Here's how the part is built. I have some questions about the finished solid (model axes, mm). Face numbers are marked on the shaded views. A direction names the side the tool comes from. Round coordinates to 2 decimals unless told otherwise and drop trailing zeros. Write each loop counter-clockwise with the first axis right and the second up, starting at its lowest first coordinate (ties: lowest second). Pieces come first, ordered by that corner, then holes. Notation, with made-up numbers: M -35,0 L 0,0 A18 ccw 0,26 Z; hole C 39,46.25 d11. An arc over 180 degrees is marked long. Use a Markdown table: item, result. Add a question column.
```python
from build123d import *

# Parameters (mm, degrees)
BOSS_EXTRUDE1_DEPTH = 80
SHELL1_T            = -3
SKETCH3_W           = 46
SKETCH3_H           = 47
BOSS_EXTRUDE2_DEPTH = 17
SKETCH4_W           = 10.2
SKETCH4_H           = 10.2
CUT_EXTRUDE1_DEPTH  = 20
SKETCH6_W           = 15
SKETCH6_H           = 12.8
CUT_EXTRUDE2_DEPTH  = 3
SKETCH7_W           = 40.4
SKETCH7_H           = 50
CUT_EXTRUDE3_DEPTH  = 5
FILLET1_R           = 4
CUT_EXTRUDE7_DEPTH  = 47
SKETCH13_R          = 1.5
CUT_EXTRUDE8_DEPTH  = 25
SKETCH14_R          = 3.1
CUT_EXTRUDE9_DEPTH  = 2
SKETCH17_W          = 45
SKETCH17_H          = 5
BOSS_EXTRUDE5_DEPTH = 74
CUT_EXTRUDE10_REACH = 126.093
SKETCH18_W          = 54
SKETCH18_H          = 45
CUT_EXTRUDE11_REACH = 126.093
SKETCH19_R          = 1.45
BOSS_EXTRUDE6_DEPTH = 47
SKETCH22_R          = 1.45
CUT_EXTRUDE12_DEPTH = 135.415364765
CUT_EXTRUDE13_REACH = 126.857
SKETCH24_R          = 3.7
SKETCH24_W          = 2
SKETCH24_H          = 3
BOSS_EXTRUDE7_DEPTH = 74
SKETCH27_R          = 1.65
CUT_EXTRUDE14_DEPTH = 10
CUT_EXTRUDE15_START = -3
CUT_EXTRUDE15_DEPTH = 32
CUT_EXTRUDE16_DEPTH = 30
BOSS_EXTRUDE8_DEPTH = 20
SKETCH31_R          = 1.5
CUT_EXTRUDE17_DEPTH = 123.649786567
CUT_EXTRUDE18_DEPTH = 15
CUT_EXTRUDE19_REACH = 126.093
SKETCH33_W          = 10
SKETCH33_H          = 5
SKETCH34_R          = 1.6
CUT_EXTRUDE20_DEPTH = 135.415364765
CUT_EXTRUDE22_DEPTH = 14
CUT_EXTRUDE23_REACH = 126.857
SKETCH37_R          = 3.2
SKETCH38_W          = 10
SKETCH38_H          = 18.980735551
SKETCH38_R          = 3.2
BOSS_EXTRUDE9_DEPTH = 3


with BuildPart() as part:
    # Sketch2 → Boss-Extrude1 (new body)
    with BuildSketch(Plane(origin=(0, 0, 0), x_dir=(0, 0, -1), z_dir=(1, 0, 0))):
        Polygon((-27.320490368, 20.998248687), (-27.320490368, -29.001751313), (12.679509632, -29.001751313), (12.679509632, -48.511383538), (27.679509632, -48.511383538), (82.679509632, 0.998248687), (82.679509632, 20.998248687), align=None)
    extrude(amount=BOSS_EXTRUDE1_DEPTH)

    # Shell1
    shell1_openings = [part.faces().sort_by_distance(p)[0] for p in [
        (40, 20.998248687, -27.679509632),
    ]]
    offset(amount=SHELL1_T, openings=shell1_openings, kind=Kind.INTERSECTION)

    # Sketch3 → Boss-Extrude2 (add)
    with BuildSketch(Plane(origin=(0, 0, 24.320490368), x_dir=(-1, 0, 0), z_dir=(0, 0, -1))):
        with Locations((-40, -2.501751313)):
            Rectangle(SKETCH3_W, SKETCH3_H)
    extrude(amount=BOSS_EXTRUDE2_DEPTH)

    # Sketch4 → Cut-Extrude1 (cut)
    with BuildSketch(Plane.XY.offset(27.320490368)):
        with Locations((40, -4.001751313)):
            Rectangle(SKETCH4_W, SKETCH4_H)
    extrude(amount=-CUT_EXTRUDE1_DEPTH, mode=Mode.SUBTRACT)

    # Sketch6 → Cut-Extrude2 (cut)
    with BuildSketch(Plane.XZ.offset(29.001751313)):
        with Locations((51.5, 0.920490368)):
            Rectangle(SKETCH6_W, SKETCH6_H)
        with Locations((28.5, 0.920490368)):
            Rectangle(SKETCH6_W, SKETCH6_H)
    extrude(amount=-CUT_EXTRUDE2_DEPTH, mode=Mode.SUBTRACT)

    # Sketch7 → Cut-Extrude3 (cut)
    with BuildSketch(Plane.XY.offset(27.320490368)):
        with Locations((40, -4.001751313)):
            Rectangle(SKETCH7_W, SKETCH7_H)
    extrude(amount=-CUT_EXTRUDE3_DEPTH, mode=Mode.SUBTRACT)

    # Fillet1
    fillet1_edges = [part.edges().sort_by_distance(p)[0] for p in [
        (19.8, -4.001751313, 27.320490368),
        (60.2, -4.001751313, 27.320490368),
        (80, -4.001751313, 27.320490368),
        (0, -4.001751313, 27.320490368),
    ]]
    fillet(fillet1_edges, radius=FILLET1_R)

    # Sketch12 → Cut-Extrude7 (cut)
    with BuildSketch(Plane(origin=(0, 20.998248687, 0), x_dir=(1, 0, 0), z_dir=(0, 1, 0))):
        Polygon((33, -7.320490368), (19.8, -12.320490368), (17, -24.320490368), (17, -7.320490368), align=None)
        Polygon((47, -7.320490368), (63, -7.320490368), (63, -24.320490368), (60.2, -12.320490368), align=None)
    extrude(amount=-CUT_EXTRUDE7_DEPTH, mode=Mode.SUBTRACT)

    # Sketch13 → Cut-Extrude8 (cut)
    with BuildSketch(Plane(origin=(0, 20.998248687, 0), x_dir=(1, 0, 0), z_dir=(0, 1, 0))):
        with Locations(Location((26, -17.320490368, 0), (0, 0, 270))):
            Circle(SKETCH13_R)
        with Locations(Location((54, -17.320490368, 0), (0, 0, 270))):
            Circle(SKETCH13_R)
    extrude(amount=-CUT_EXTRUDE8_DEPTH, mode=Mode.SUBTRACT)

    # Sketch14 → Cut-Extrude9 (cut)
    with BuildSketch(Plane(origin=(0, 20.998248687, 0), x_dir=(1, 0, 0), z_dir=(0, 1, 0))):
        with Locations(Location((26, -17.320490368, 0), (0, 0, 270))):
            Circle(SKETCH14_R)
        with Locations(Location((54, -17.320490368, 0), (0, 0, 270))):
            Circle(SKETCH14_R)
    extrude(amount=-CUT_EXTRUDE9_DEPTH, mode=Mode.SUBTRACT)

    # Sketch17 → Boss-Extrude5 (add)
    with BuildSketch(Plane.ZY.offset(-77)):
        with Locations((-23.179509632, -4.501751313)):
            Rectangle(SKETCH17_W, SKETCH17_H)
    extrude(amount=BOSS_EXTRUDE5_DEPTH)

    # Sketch18 → Cut-Extrude10 (cut, up to next)
    with BuildSketch(Plane(origin=(0, -2.001751313, 0), x_dir=(1, 0, 0), z_dir=(0, 1, 0)), mode=Mode.PRIVATE) as cut_extrude10_sk1:
        with Locations((40, 23.179509632)):
            Rectangle(SKETCH18_W, SKETCH18_H)
    cut_extrude10_tool1 = extrude(cut_extrude10_sk1.sketch, amount=-CUT_EXTRUDE10_REACH, mode=Mode.PRIVATE) & part.part
    add(cut_extrude10_tool1.solids().sort_by_distance((40, -2.001751, -23.17951))[0], mode=Mode.SUBTRACT)

    # Sketch19 → Cut-Extrude11 (cut, up to next)
    with BuildSketch(Plane(origin=(0, -2.001751313, 0), x_dir=(1, 0, 0), z_dir=(0, 1, 0)), mode=Mode.PRIVATE) as cut_extrude11_sk1:
        with Locations(Location((72, 37.179509632, 0), (0, 0, 270))):
            Circle(SKETCH19_R)
    cut_extrude11_tool1 = extrude(cut_extrude11_sk1.sketch, amount=-CUT_EXTRUDE11_REACH, mode=Mode.PRIVATE) & part.part
    # Sketch19 → Cut-Extrude11 (cut, up to next)
    with BuildSketch(Plane(origin=(0, -2.001751313, 0), x_dir=(1, 0, 0), z_dir=(0, 1, 0)), mode=Mode.PRIVATE) as cut_extrude11_sk2:
        with Locations(Location((72, 6.179509632, 0), (0, 0, 270))):
            Circle(SKETCH19_R)
    cut_extrude11_tool2 = extrude(cut_extrude11_sk2.sketch, amount=-CUT_EXTRUDE11_REACH, mode=Mode.PRIVATE) & part.part
    # Sketch19 → Cut-Extrude11 (cut, up to next)
    with BuildSketch(Plane(origin=(0, -2.001751313, 0), x_dir=(1, 0, 0), z_dir=(0, 1, 0)), mode=Mode.PRIVATE) as cut_extrude11_sk3:
        with Locations(Location((8, 33.179509632, 0), (0, 0, 270))):
            Circle(SKETCH19_R)
    cut_extrude11_tool3 = extrude(cut_extrude11_sk3.sketch, amount=-CUT_EXTRUDE11_REACH, mode=Mode.PRIVATE) & part.part
    # Sketch19 → Cut-Extrude11 (cut, up to next)
    with BuildSketch(Plane(origin=(0, -2.001751313, 0), x_dir=(1, 0, 0), z_dir=(0, 1, 0)), mode=Mode.PRIVATE) as cut_extrude11_sk4:
        with Locations(Location((8, 6.179509632, 0), (0, 0, 270))):
            Circle(SKETCH19_R)
    cut_extrude11_tool4 = extrude(cut_extrude11_sk4.sketch, amount=-CUT_EXTRUDE11_REACH, mode=Mode.PRIVATE) & part.part
    add(cut_extrude11_tool1.solids().sort_by_distance((72, -2.001751, -37.17951))[0], mode=Mode.SUBTRACT)
    add(cut_extrude11_tool2.solids().sort_by_distance((72, -2.001751, -6.17951))[0], mode=Mode.SUBTRACT)
    add(cut_extrude11_tool3.solids().sort_by_distance((8, -2.001751, -33.17951))[0], mode=Mode.SUBTRACT)
    add(cut_extrude11_tool4.solids().sort_by_distance((8, -2.001751, -6.17951))[0], mode=Mode.SUBTRACT)

    # Sketch21 → Boss-Extrude6 (add)
    with BuildSketch(Plane(origin=(0, -26.001751313, 0), x_dir=(1, 0, 0), z_dir=(0, 1, 0))):
        Polygon((3, -24.320490368), (3, -14.320490368), (19.333333333, -14.320490368), (17, -24.320490368), align=None)
    extrude(amount=BOSS_EXTRUDE6_DEPTH)

    # Sketch22 → Cut-Extrude12 (cut, through all)
    with BuildSketch(Plane(origin=(0, 20.998248687, 0), x_dir=(1, 0, 0), z_dir=(0, 1, 0))):
        with Locations(Location((10, -19.320490368, 0), (0, 0, 270))):
            Circle(SKETCH22_R)
    extrude(amount=-CUT_EXTRUDE12_DEPTH, mode=Mode.SUBTRACT)

    # Sketch24 → Cut-Extrude13 (cut, up to next)
    with BuildSketch(Plane(origin=(80, 0, 0), x_dir=(0, 0, -1), z_dir=(1, 0, 0)), mode=Mode.PRIVATE) as cut_extrude13_sk1:
        with Locations((26.679509632, -30.511383538)):
            Circle(SKETCH24_R)
    cut_extrude13_tool1 = extrude(cut_extrude13_sk1.sketch, amount=-CUT_EXTRUDE13_REACH, mode=Mode.PRIVATE) & part.part
    # Sketch24 → Cut-Extrude13 (cut, up to next)
    with BuildSketch(Plane(origin=(80, 0, 0), x_dir=(0, 0, -1), z_dir=(1, 0, 0)), mode=Mode.PRIVATE) as cut_extrude13_sk2:
        with Locations((34.379509632, -30.511383538)):
            Rectangle(SKETCH24_W, SKETCH24_H)
    cut_extrude13_tool2 = extrude(cut_extrude13_sk2.sketch, amount=-CUT_EXTRUDE13_REACH, mode=Mode.PRIVATE) & part.part
    add(cut_extrude13_tool1.solids().sort_by_distance((80, -30.511384, -26.67951))[0], mode=Mode.SUBTRACT)
    add(cut_extrude13_tool2.solids().sort_by_distance((80, -30.511384, -34.37951))[0], mode=Mode.SUBTRACT)

    # Sketch26 → Boss-Extrude7 (add)
    with BuildSketch(Plane(origin=(3, 0, 0), x_dir=(0, 0, -1), z_dir=(1, 0, 0))):
        Polygon((79.679509632, 2.334161996), (63.679509632, 2.334161996), (63.679509632, -12.068640106), align=None)
    extrude(amount=BOSS_EXTRUDE7_DEPTH)

    # Sketch27 → Cut-Extrude14 (cut)
    with BuildSketch(Plane(origin=(0, 2.334161996, 0), x_dir=(1, 0, 0), z_dir=(0, 1, 0))):
        with Locations(Location((6, 76.679509632, 0), (0, 0, 270))):
            Circle(SKETCH27_R)
        with Locations(Location((74, 76.679509632, 0), (0, 0, 270))):
            Circle(SKETCH27_R)
    extrude(amount=-CUT_EXTRUDE14_DEPTH, mode=Mode.SUBTRACT)

    # Sketch28 → Cut-Extrude15 (cut)
    with BuildSketch(Plane(origin=(0, 2.334161996, 0), x_dir=(1, 0, 0), z_dir=(0, 1, 0)).offset(CUT_EXTRUDE15_START)):
        Polygon((74, 79.929509632), (71.185417438, 78.304509632), (71.185417438, 75.054509632), (74, 73.429509632), (76.814582562, 75.054509632), (76.814582562, 78.304509632), align=None)
        Polygon((6, 73.429509632), (8.814582562, 75.054509632), (8.814582562, 78.304509632), (6, 79.929509632), (3.185417438, 78.304509632), (3.185417438, 75.054509632), align=None)
    extrude(amount=-CUT_EXTRUDE15_DEPTH, mode=Mode.SUBTRACT)

    # Sketch29 → Cut-Extrude16 (cut)
    with BuildSketch(Plane.XZ.offset(29.001751313)):
        Polygon((7.185417438, 17.695490368), (10, 16.070490368), (12.814582562, 17.695490368), (12.814582562, 20.945490368), (10, 22.570490368), (7.185417438, 20.945490368), align=None)
    extrude(amount=-CUT_EXTRUDE16_DEPTH, mode=Mode.SUBTRACT)

    # Sketch30 → Boss-Extrude8 (add)
    with BuildSketch(Plane(origin=(0, -26.001751313, 0), x_dir=(1, 0, 0), z_dir=(0, 1, 0))):
        Polygon((77, -24.320490368), (63, -24.320490368), (60.2, -12.320490368), (77, -12.320490368), align=None)
    extrude(amount=BOSS_EXTRUDE8_DEPTH)

    # Sketch31 → Cut-Extrude17 (cut, through all)
    with BuildSketch(Plane(origin=(0, -6.001751313, 0), x_dir=(1, 0, 0), z_dir=(0, 1, 0))):
        with Locations(Location((72, -21.320490368, 0), (0, 0, 270))):
            Circle(SKETCH31_R)
    extrude(amount=-CUT_EXTRUDE17_DEPTH, mode=Mode.SUBTRACT)

    # Sketch32 → Cut-Extrude18 (cut)
    with BuildSketch(Plane.XZ.offset(29.001751313)):
        Polygon((72, 24.570490368), (69.185417438, 22.945490368), (69.185417438, 19.695490368), (72, 18.070490368), (74.814582562, 19.695490368), (74.814582562, 22.945490368), align=None)
    extrude(amount=-CUT_EXTRUDE18_DEPTH, mode=Mode.SUBTRACT)

    # Sketch33 → Cut-Extrude19 (cut, up to next)
    with BuildSketch(Plane(origin=(0, -2.001751313, 0), x_dir=(1, 0, 0), z_dir=(0, 1, 0)), mode=Mode.PRIVATE) as cut_extrude19_sk1:
        with Locations((72, 43.179509632)):
            Rectangle(SKETCH33_W, SKETCH33_H)
    cut_extrude19_tool1 = extrude(cut_extrude19_sk1.sketch, amount=-CUT_EXTRUDE19_REACH, mode=Mode.PRIVATE) & part.part
    add(cut_extrude19_tool1.solids().sort_by_distance((72, -2.001751, -43.17951))[0], mode=Mode.SUBTRACT)

    # Sketch34 → Cut-Extrude20 (cut, through all)
    with BuildSketch(Plane(origin=(0, 20.998248687, 0), x_dir=(1, 0, 0), z_dir=(0, 1, 0))):
        with Locations(Location((40, -17.320490368, 0), (0, 0, 270))):
            Circle(SKETCH34_R)
    extrude(amount=-CUT_EXTRUDE20_DEPTH, mode=Mode.SUBTRACT)

    # Sketch36 → Cut-Extrude22 (cut)
    with BuildSketch(Plane.XZ.offset(29.001751313)):
        Polygon((38.375, 20.13507293), (36.75, 17.320490368), (38.375, 14.505907805), (41.625, 14.505907805), (43.25, 17.320490368), (41.625, 20.13507293), align=None)
    extrude(amount=-CUT_EXTRUDE22_DEPTH, mode=Mode.SUBTRACT)

    # Sketch37 → Cut-Extrude23 (cut, up to next)
    with BuildSketch(Plane(origin=(80, 0, 0), x_dir=(0, 0, -1), z_dir=(1, 0, 0)), mode=Mode.PRIVATE) as cut_extrude23_sk1:
        with Locations((-3.320490368, -16.511383538)):
            Circle(SKETCH37_R)
    cut_extrude23_tool1 = extrude(cut_extrude23_sk1.sketch, amount=-CUT_EXTRUDE23_REACH, mode=Mode.PRIVATE) & part.part
    add(cut_extrude23_tool1.solids().sort_by_distance((80, -16.511384, 3.32049))[0], mode=Mode.SUBTRACT)

    # Sketch38 → Boss-Extrude9 (add)
    with BuildSketch(Plane.ZY.offset(-77)):
        with Locations((3.320490368, -16.511383538)):
            Rectangle(SKETCH38_W, SKETCH38_H)
        with Locations(Location((3.320490368, -16.511383538, 0), (0, 0, 180))):
            Circle(SKETCH38_R, mode=Mode.SUBTRACT)
    extrude(amount=BOSS_EXTRUDE9_DEPTH)


solid = part.part
```
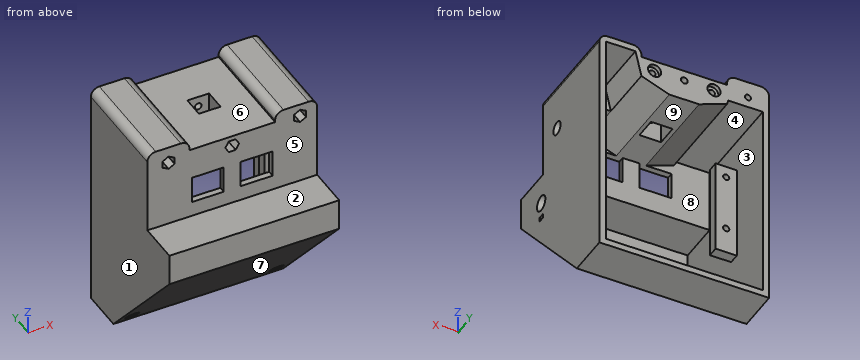
Item 1: Imagine slicing it at B-B on x = 26. List the corners of the cut face in (y, z) for me.
Item 2: Imagine slicing it at A-A on z = -3. List the corners of the cut face in (x, y) for me, plus the area to 3 significant figures.
Item 3: Imagine slicing it at C-C on y = 16. List the corners of the cut face in (x, z) for me.
Item 4: Imagine slicing it at D-D on x = 40. Count the separate pieces of the cut face and the enclosed holes in it, plus the area to 3 significant figures.
Item 5: For pin 1 Ø18.5 at (x, y) = (72.5, -12.5) entering from -Z; pin 2 Ø5 at (x, y) = (39.5, -27.5) entering from -Z; pin 3 Ø1.7 at (x, z) = (73.5, -75.5) entering from -Y; pin 4 Ø3 at (y, z) = (-29, -54.5) entering from +X, each with a flat end and sliding along its axis, tell me the tip position at first contact or that it passes through.
Item 6: On a 3-axis mill with a long thin cutter (end or side, diameter ignored), from which of +Z, -Z, +X, -X, +Y, -Y can I reach the whole of each face in a straight line? I mean the marked faces 5, 6, 7, 8 and 9. Say none if no direction works.
Item 7: If we mould it in two halves opening along X, with no side actions, what happens to the marked faces 1, 2, 3 and 4? For each: +X half, -X half, draft (parallel to the pull), parting line (faces both ways), or undercut.
Item 8: I need wall thicknesses on probe 1 along X at (y, z) = (11, -8); probe 2 along Z at (x, y) = (5, 3); probe 3 along X at (y, z) = (-8.5, 15). Which ranges of each line are inside material? Lowest first, please. Write a range as from..to.
The answers:
| question | item | result |
|---|---|---|
| 1 | outline | M -48.51,-27.68 L 1,-82.68 L 21,-82.68 L 21,-79.68 L 2.33,-79.68 L 2.33,-63.68 L -12.07,-63.68 L -45.51,-26.53 L -45.51,-15.68 L -26,-15.68 L -26,-5.48 L -29,-5.48 L -29,-12.68 L -48.51,-12.68 Z; M -29,7.32 L -26,7.32 L -26,9.97 L 21,9.97 L 21,14.22 L 19,14.22 L 19,15.82 L -4,15.82 L -4,18.82 L 19,18.82 L 19,20.42 L 21,20.42 L 21,22.32 L -29,22.32 Z |
| 2 | outline | M 0,-29 L 21,-29 L 21,-26 L 3,-26 L 3,-7 L 13,-7 L 13,-2 L 3,-2 L 3,21 L 0,21 Z; M 36,-29 L 44,-29 L 44,-26 L 36,-26 Z; M 59,-29 L 80,-29 L 80,21 L 77,21 L 77,-2 L 67,-2 L 67,-7 L 77,-7 L 77,-26 L 59,-26 Z |
| 2 | area | 532 mm² |
| 3 | outline | M 0,-82.68 L 80,-82.68 L 80,23.32 A4 ccw 76,27.32 L 64.2,27.32 A4 ccw 60.2,23.32 L 60.2,22.32 L 19.8,22.32 L 19.8,23.32 A4 ccw 15.8,27.32 L 4,27.32 A4 ccw 0,23.32 Z; hole M 3,-79.68 L 77,-79.68 L 77,24.32 L 63,24.32 L 60.2,12.32 L 47,7.32 L 33,7.32 L 19.8,12.32 L 19.33,14.32 L 3,14.32 Z; hole C 10,19.32 d2.9; hole C 26,17.32 d3; hole C 40,17.32 d3.2; hole C 54,17.32 d3 |
| 4 | separate pieces | 4 |
| 4 | enclosed holes | 0 |
| 4 | area | 989 mm² |
| 5 | pin 1 | z = -77.86 |
| 5 | pin 2 | z = -53.8 |
| 5 | pin 3 | y = -0.67 |
| 5 | pin 4 | through |
| 6 | face 5 | +Z, +X, -X, -Y |
| 6 | face 6 | +Z, +Y, -Y |
| 6 | face 7 | -Z, +X, -X, -Y |
| 6 | face 8 | none |
| 6 | face 9 | +Y |
| 7 | face 1 | -X half |
| 7 | face 2 | draft |
| 7 | face 3 | undercut |
| 7 | face 4 | undercut |
| 8 | probe 1 | 0..3, 77..80 |
| 8 | probe 2 | -82.68..-79.68, 14.32..27.32 |
| 8 | probe 3 | 0..34.9, 45.1..80 |
